The model under review builds one solid part; all positions refer to its coordinate system, in mm. Round coordinates to 2 decimals unless told otherwise and drop trailing zeros. Order: outer loops, then holes, each group sorted by start corner. A loop starts at its lowest first (then second) coordinate and runs counter-clockwise, first axis right, second up.
```python
from build123d import *

# Parameters (mm, degrees)
SKETCH_1_R      = 15.5
SKETCH_1_R_2    = 9
SKETCH_1_R_3    = 2.5
SKETCH_1_R_4    = 1.6
EXTRUDE_1_DEPTH = 1.5


with BuildPart() as part:
    # Эскиз1 → Бобышка-Вытянуть1 (new body)
    with BuildSketch(Plane.XY):
        Circle(SKETCH_1_R)
        with Locations((-5, 0)):
            Circle(SKETCH_1_R_2, mode=Mode.SUBTRACT)
        with Locations((9.6, 0)):
            Circle(SKETCH_1_R_3, mode=Mode.SUBTRACT)
        with Locations((0, 10)):
            Circle(SKETCH_1_R_4, mode=Mode.SUBTRACT)
        with Locations(Location((0, -10, 0), (0, 0, 180))):
            Circle(SKETCH_1_R_4, mode=Mode.SUBTRACT)
    extrude(amount=EXTRUDE_1_DEPTH)


solid = part.part
```
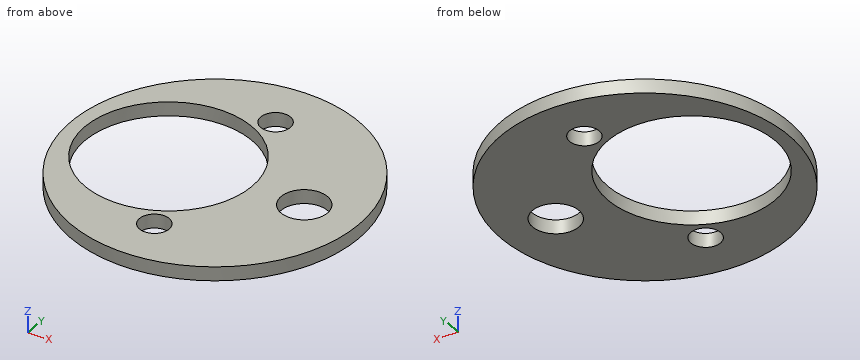
(1) Consider section C-C (x = -8). Write out the cut boundary in (y, z).
Data:
outline: (-13.28, 0) - (-8.49, 0) - (-8.49, 1.5) - (-13.28, 1.5) - close; (8.49, 0) - (13.28, 0) - (13.28, 1.5) - (8.49, 1.5) - close
(2) Consider section A-A (y = 0). Write out the cut boundary in (x, z), and give its area (3 significant figures).
Data:
outline: (-15.5, 0) - (-14, 0) - (-14, 1.5) - (-15.5, 1.5) - close; (4, 0) - (7.1, 0) - (7.1, 1.5) - (4, 1.5) - close; (12.1, 0) - (15.5, 0) - (15.5, 1.5) - (12.1, 1.5) - close
area: 12.0 mm2
(3) Consider section B-B (z = 1). Write out the cut boundary in (x, y), and give its area (3 significant figures).
Data:
outline: circle Ø31 at (0, 0); hole circle Ø18 at (-5, 0); hole circle Ø3.2 at (0, -10); hole circle Ø3.2 at (0, 10); hole circle Ø5 at (9.6, 0)
area: 465 mm2
(4) Consider section D-D (y = 6.5). Write out the cut boundary in (x, z), and give its area (3 significant figures).
Data:
outline: (-14.07, 0) - (-11.22, 0) - (-11.22, 1.5) - (-14.07, 1.5) - close; (1.22, 0) - (14.07, 0) - (14.07, 1.5) - (1.22, 1.5) - close
area: 23.5 mm2
(5) Insertion check: pin 1 (4.5 mm diameter, centred on x = 9.6, y = 0, fed in from -Z); pin 2 (3.5 mm diameter, centred on x = 0, y = -10, fed in from +Z). Each pin has a flat end and moves straight along its axis. Give the tip position at first contact, or say it passes through.
Data:
pin 1: passes through
pin 2: stops at z = 1.5
(6) To check wall thickness, follow probe 1 along Y at (x, z) = (1, 0.3); probe 2 along Y at (x, z) = (0, 0.9); probe 3 along X at (y, z) = (1, 0.5). State the ranges of each line that lie inside material, in increasing order.
Data:
probe 1: y = -15.47 to -11.25, -8.75 to -6.71, 6.71 to 8.75, 11.25 to 15.47
probe 2: y = -15.5 to -11.6, -8.4 to -7.48, 7.48 to 8.4, 11.6 to 15.5
probe 3: x = -15.47 to -13.94, 3.94 to 7.31, 11.89 to 15.47
